Design review of the part built by this model. Coordinates are the model's own, in mm. Round coordinates to 2 decimals unless told otherwise and drop trailing zeros. Loops run counter-clockwise (first coordinate to the right, second up) from the corner with the lowest first, then second, coordinate; pieces in that order, holes last. Notation, with made-up numbers: M 12.5,67 L 61.5,67 A13 cw 61.5,75 Z; hole C 88,-23.75 d9. An arc over 180 degrees is marked long. One line per item, written item: value. Start each with the question number.
Item 1: We need section B-B (x = 2.65). Write out the cut boundary in (y, z).
Item 2: We need section A-A (z = -601.5). Write out the cut boundary in (x, y).
Item 3: We need section D-D (y = 148). Write out the cut boundary in (x, z).
Item 4: For line 1 along Y through (x, z) = (4, -491); line 2 along Y through (x, z) = (2.25, -507); line 3 along Y through (x, z) = (0.95, -451), list the stretches that pass through material, from the lowest coordinate up.
Item 5: We need section C-C (z = -542.5). Write out the cut boundary in (x, y).
from build123d import *

# Parameters (mm, degrees)
F1_DEPTH = 4.5


# Not quite as in the source:
# - a feature names something its author has since deleted; it is built from what else it names


with BuildPart() as f1:
    # F0 (on Right) → F1 (new body)
    with BuildSketch(Plane.YZ):
        with BuildLine():
            Line((-100, -666.4014723765), (294.8394132124, -666.4014723765))
            Line((294.8394132124, -666.4014723765), (294.8394132124, -466.4014723765))
            ThreePointArc((294.8394132124, -466.4014723765), (277.2658200836, -423.9750655053), (234.8394132124, -406.4014723765))
            Line((234.8394132124, -406.4014723765), (-460.1605867876, -406.4014723765))
            ThreePointArc((-460.1605867876, -406.4014723765), (-491.980391941, -419.5816672231), (-505.1605867876, -451.4014723765))
            Line((-505.1605867876, -451.4014723765), (-505.1605867876, -666.4014723765))
            Line((-505.1605867876, -666.4014723765), (-100, -666.4014723765))
        make_face()
        with BuildLine():
            ThreePointArc((-24.6605867876, -611.4014723765), (-35.1605867876, -621.9014723765), (-45.6605867876, -611.4014723765))
            Line((-45.6605867876, -611.4014723765), (-45.6605867876, -511.4014723765))
            ThreePointArc((-45.6605867876, -511.4014723765), (-35.1605867876, -500.9014723765), (-24.6605867876, -511.4014723765))
            Line((-24.6605867876, -511.4014723765), (-24.6605867876, -611.4014723765))
        make_face(mode=Mode.SUBTRACT)
        with BuildLine():
            ThreePointArc((-453.1605867876, -611.4014723765), (-463.6605867876, -621.9014723765), (-474.1605867876, -611.4014723765))
            Line((-474.1605867876, -611.4014723765), (-474.1605867876, -451.4014723765))
            ThreePointArc((-474.1605867876, -451.4014723765), (-463.6605867876, -440.9014723765), (-453.1605867876, -451.4014723765))
            Line((-453.1605867876, -451.4014723765), (-453.1605867876, -611.4014723765))
        make_face(mode=Mode.SUBTRACT)
        with BuildLine():
            Line((34.3394132124, -611.4014723765), (34.3394132124, -451.4014723765))
            ThreePointArc((34.3394132124, -451.4014723765), (44.8394132124, -440.9014723765), (55.3394132124, -451.4014723765))
            Line((55.3394132124, -451.4014723765), (55.3394132124, -611.4014723765))
            ThreePointArc((55.3394132124, -611.4014723765), (44.8394132124, -621.9014723765), (34.3394132124, -611.4014723765))
        make_face(mode=Mode.SUBTRACT)
        with BuildLine():
            Line((134.3394132124, -611.4014723765), (134.3394132124, -451.4014723765))
            ThreePointArc((134.3394132124, -451.4014723765), (144.8394132124, -440.9014723765), (155.3394132124, -451.4014723765))
            Line((155.3394132124, -451.4014723765), (155.3394132124, -611.4014723765))
            ThreePointArc((155.3394132124, -611.4014723765), (144.8394132124, -621.9014723765), (134.3394132124, -611.4014723765))
        make_face(mode=Mode.SUBTRACT)
        with BuildLine():
            ThreePointArc((235.3394132124, -581.4014723765), (224.8394132124, -591.9014723765), (214.3394132124, -581.4014723765))
            Line((214.3394132124, -581.4014723765), (214.3394132124, -481.4014723765))
            ThreePointArc((214.3394132124, -481.4014723765), (224.8394132124, -470.9014723765), (235.3394132124, -481.4014723765))
            Line((235.3394132124, -481.4014723765), (235.3394132124, -581.4014723765))
        make_face(mode=Mode.SUBTRACT)
    extrude(amount=F1_DEPTH)


solid = f1.part
A:
1. outline: M -505.16,-666.4 L 294.84,-666.4 L 294.84,-466.4 A60 ccw 234.84,-406.4 L -460.16,-406.4 A45 ccw -505.16,-451.4 Z; hole M -474.16,-611.4 A10.5 ccw -453.16,-611.4 L -453.16,-451.4 A10.5 ccw -474.16,-451.4 Z; hole M -45.66,-611.4 A10.5 ccw -24.66,-611.4 L -24.66,-511.4 A10.5 ccw -45.66,-511.4 Z; hole M 34.34,-611.4 A10.5 ccw 55.34,-611.4 L 55.34,-451.4 A10.5 ccw 34.34,-451.4 Z; hole M 134.34,-611.4 A10.5 ccw 155.34,-611.4 L 155.34,-451.4 A10.5 ccw 134.34,-451.4 Z; hole M 214.34,-581.4 A10.5 ccw 235.34,-581.4 L 235.34,-481.4 A10.5 ccw 214.34,-481.4 Z
2. outline: M 0,-505.16 L 4.5,-505.16 L 4.5,-474.16 L 0,-474.16 Z; M 0,-453.16 L 4.5,-453.16 L 4.5,-45.66 L 0,-45.66 Z; M 0,-24.66 L 4.5,-24.66 L 4.5,34.34 L 0,34.34 Z; M 0,55.34 L 4.5,55.34 L 4.5,134.34 L 0,134.34 Z; M 0,155.34 L 4.5,155.34 L 4.5,294.84 L 0,294.84 Z
3. outline: M 0,-666.4 L 4.5,-666.4 L 4.5,-621.41 L 0,-621.41 Z; M 0,-441.39 L 4.5,-441.39 L 4.5,-406.4 L 0,-406.4 Z
4. line 1: -505.16 to -474.16, -453.16 to 34.34, 55.34 to 134.34, 155.34 to 214.34, 235.34 to 294.84
4. line 2: -505.16 to -474.16, -453.16 to -44.69, -25.63 to 34.34, 55.34 to 134.34, 155.34 to 214.34, 235.34 to 294.84
4. line 3: -505.16 to -474.15, -453.17 to 34.35, 55.33 to 134.35, 155.33 to 292.83
5. outline: M 0,-505.16 L 4.5,-505.16 L 4.5,-474.16 L 0,-474.16 Z; M 0,-453.16 L 4.5,-453.16 L 4.5,-45.66 L 0,-45.66 Z; M 0,-24.66 L 4.5,-24.66 L 4.5,34.34 L 0,34.34 Z; M 0,55.34 L 4.5,55.34 L 4.5,134.34 L 0,134.34 Z; M 0,155.34 L 4.5,155.34 L 4.5,214.34 L 0,214.34 Z; M 0,235.34 L 4.5,235.34 L 4.5,294.84 L 0,294.84 Z
